```python
from build123d import *

# Parameters (mm, degrees)
F0_R     = 16.5
F1_DEPTH = 945
F3_DEPTH = 500
F5_DEPTH = 50


with BuildPart() as f1:
    # F0 (on Front) → F1 (new body)
    with BuildSketch(Plane.XZ):
        Circle(F0_R)
    extrude(amount=F1_DEPTH)

    # F2 (on Top) → F3 (cut, symmetric)
    with BuildSketch(Plane.XY):
        with BuildLine():
            Line((0, 0), (-21, 0))
            ThreePointArc((-21, 0), (0, -16.890228), (21, 0))
            Line((21, 0), (0, 0))
        make_face()
    extrude(amount=F3_DEPTH, both=True, mode=Mode.SUBTRACT)

    # F4 (on Top) → F5 (cut, symmetric)
    with BuildSketch(Plane.XY):
        with BuildLine():
            Line((-21, -945), (21, -945))
            ThreePointArc((21, -945), (0, -924), (-21, -945))
        make_face()
    extrude(amount=F5_DEPTH, both=True, mode=Mode.SUBTRACT)


solid = f1.part
```
Work out the finished part from the listing and answer in its coordinate system (mm). Coordinates: 2 decimals unless noted, no trailing zeros. Loops run counter-clockwise (first coordinate to the right, second up) from the corner with the lowest first, then second, coordinate; pieces in that order, holes last.
1) Section C-C (z = 9) is taken. Give the vertices of the cut face in (x, y).
Results:
outline: (-13.83, -929.2) arc R21 cw to (13.83, -929.2) - (13.83, -11.85) arc R21.5 cw to (-13.83, -11.85) - close
2) Section B-B (x = -8.5) is taken. Give the vertices of the cut face in (y, z), plus the area to 3 significant figures.
Results:
outline: (-925.8, -14.14) - (-15.14, -14.14) - (-15.14, 14.14) - (-925.8, 14.14) - close
area: 25,800 mm2
3) Section A-A (y = -641) is taken. Give the vertices of the cut face in (x, z).
Results:
outline: circle Ø33 at (0, 0)
4) Flat-ended cylindrical pins translate along their axes: pin 1 (4 mm diameter, centred on x = 12, z = 5, fed in from +Y); pin 2 (1.5 mm diameter, centred on x = -11, z = -0.5, fed in from +Y); pin 3 (1 mm diameter, centred on y = -172, z = 1, fed in from -X). Find the tip coordinate at first contact, or state that the pin passes through.
Results:
pin 1: stops at y = -11.71
pin 2: stops at y = -13.4
pin 3: stops at x = -16.49
5) Consider probe 1 along X at (y, z) = (-403.5, -2); probe 2 along Y at (x, z) = (0.5, 12.5); probe 3 along Z at (x, y) = (-15, -334). Determine where each line is inside the solid, lowest interval first.
Results:
probe 1: x = -16.38 to 16.38
probe 2: y = -924.01 to -16.88
probe 3: z = -6.87 to 6.87
6) For a pull along X with two mould halves and no side action, classify faces 1 (the cylindrical face through (15.24, -464.13, -6.32)), 2 (the cylindrical face through (0, -924, 0)) as +X half, -X half, draft (parallel to the pull), parting line (faces both ways), or undercut.
Results:
face 1: parting line
face 2: undercut
